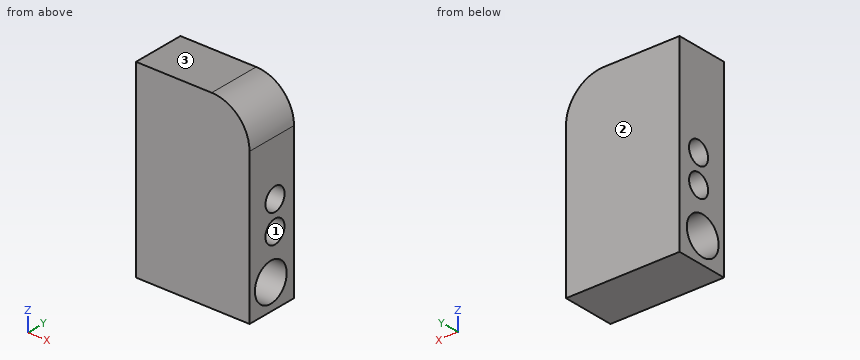
from build123d import *

# Parameters (mm, degrees)
F1_DEPTH = 7
F2_R     = 1.5
F2_R_2   = 2.5
F3_DEPTH = 20


with BuildPart() as f1:
    # F0 (on Front) → F1 (new body)
    with BuildSketch(Plane.XZ):
        with BuildLine():
            Line((10, 0), (0, 0))
            Line((0, 0), (0, -25))
            Line((0, -25), (15, -25))
            Line((15, -25), (15, -5))
            ThreePointArc((15, -5), (13.535534, -1.464466), (10, 0))
        make_face()
    extrude(amount=F1_DEPTH)

    # F2 (on face) → F3 (cut)
    with BuildSketch(Plane(origin=(0, 0, 0), x_dir=(0, -1, 0), z_dir=(-1, 0, 0))):
        with Locations((2.988549, -12.238131)):
            Circle(F2_R)
        with Locations((3, -16)):
            Circle(F2_R)
        with Locations((3.653436, -21.588029)):
            Circle(F2_R_2)
    extrude(amount=-F3_DEPTH, mode=Mode.SUBTRACT)


solid = f1.part
Could you check a few things on this model? Use its own coordinates, in mm. Face numbers are marked on the shaded views. Give positions to 0.01 mm unless a question says otherwise; leave off trailing zeros. Write each loop counter-clockwise with the first axis right and the second up, starting at its lowest first coordinate (ties: lowest second). Pieces come first, ordered by that corner, then holes. Notation, with made-up numbers: (38.25, 46.5) -> (73.25, 46.5) arc R9 cw to (73.25, 50.5) -> close; hole circle Ø8 at (-16, 13.5). An arc over 180 degrees is marked (long way). Write each question's results on one line, items separated by ' | '. Start each with the question number.
Q1. Suppose I cut it at B-B, the plane y = -5.25. List the corners of the cut face in (x, z) for me.
Q2. Suppose I cut it at A-A, the plane z = -16. List the corners of the cut face in (x, y) for me, and give its area (3 significant figures).
Q3. I'm going to push a flat-ended pin straight in: pin 1 Ø2.5 at (y, z) = (-2.99, -12.24) entering from +X. Where does the tip first touch, or does it pass through?
Q4. We'd pull the mould along Y, two halves only. Please class the marked faces 1, 2 and 3: +Y half, -Y half, draft (parallel to the pull), parting line (faces both ways), or undercut.
Q5. Suppose I cut it at C-C, the plane x = 11. List the corners of the cut face in (y, z) for me.
Q6. Suppose I cut it at D-D, the plane y = -3. List the corners of the cut face in (x, z) for me.
Q7. I need wall thicknesses on probe 1 along Y at (x, z) = (7.25, -21.5); probe 2 along Z at (x, y) = (13, -1.75); probe 3 along Y at (x, z) = (8, -21.75). Which ranges of each line are inside material? Lowest first, please.
Outcome:
1) outline: (0, -25) -> (15, -25) -> (15, -23.51) -> (0, -23.51) -> close; (0, -19.66) -> (15, -19.66) -> (15, -5) arc R5 ccw to (10, 0) -> (0, 0) -> close
2) outline: (0, -7) -> (15, -7) -> (15, -4.5) -> (0, -4.5) -> close; (0, -1.5) -> (15, -1.5) -> (15, 0) -> (0, 0) -> close | area: 60.0 mm2
3) pin 1: through
4) face 1: undercut | face 2: +Y half | face 3: draft
5) outline: (-7, -25) -> (0, -25) -> (0, -0.1) -> (-7, -0.1) -> close; hole circle Ø5 at (-3.65, -21.59); hole circle Ø3 at (-3, -16); hole circle Ø3 at (-2.99, -12.24)
6) outline: (0, -25) -> (15, -25) -> (15, -24) -> (0, -24) -> close; (0, -19.17) -> (15, -19.17) -> (15, -17.5) -> (0, -17.5) -> close; (0, -14.5) -> (15, -14.5) -> (15, -13.74) -> (0, -13.74) -> close; (0, -10.74) -> (15, -10.74) -> (15, -5) arc R5 ccw to (10, 0) -> (0, 0) -> close
7) probe 1: -7 to -6.15, -1.15 to 0 | probe 2: -25 to -23.21, -19.97 to -16.83, -15.17 to -13.08, -11.39 to -1 | probe 3: -7 to -6.15, -1.16 to 0
